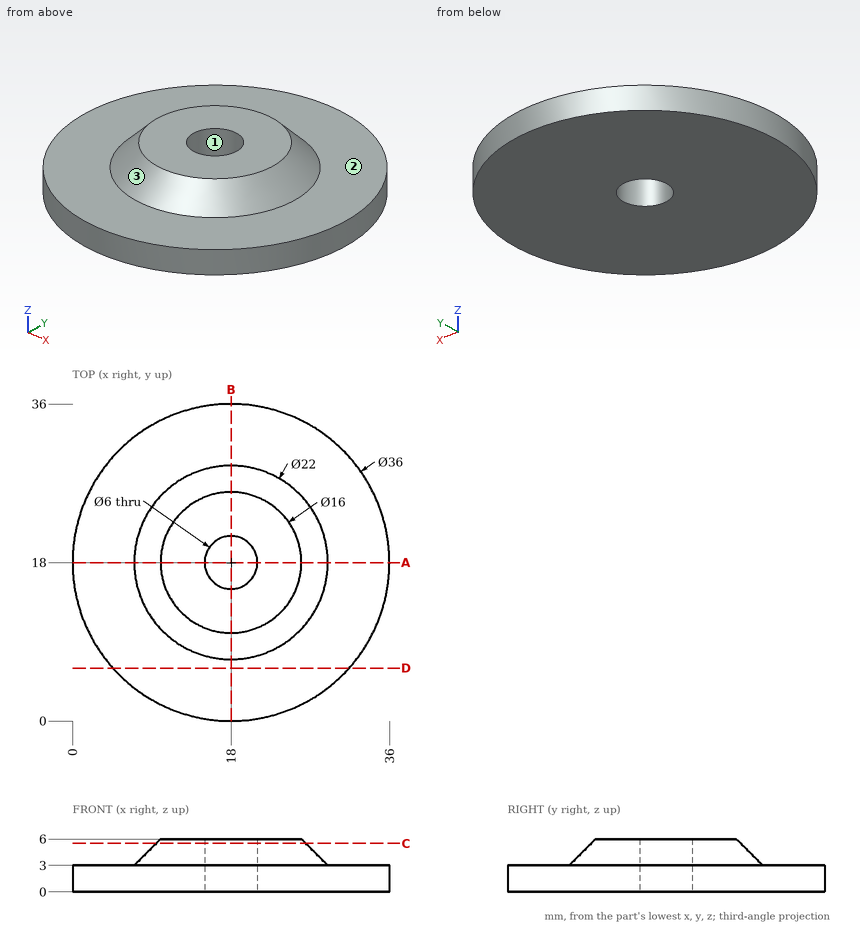
Input: dimensioned drawing with shaded views. Units: mm. Origin: part minimum x, y, z. Coordinates: 2 decimals unless noted, no trailing zeros. Loops run counter-clockwise (first coordinate to the right, second up) from the corner with the lowest first, then second, coordinate; pieces in that order, holes last.
Q1. Section A-A, the plane y = 18. Return the cut outline in (x, z).
Results are:
outline: (0, 0) - (15, 0) - (15, 6) - (10, 6) - (7, 3) - (0, 3) - close; (21, 0) - (36, 0) - (36, 3) - (29, 3) - (26, 6) - (21, 6) - close
Q2. Section D-D, the plane y = 6. Return the cut outline in (x, z), and give its area (3 significant figures).
Results are:
outline: (4.58, 0) - (31.42, 0) - (31.42, 3) - (4.58, 3) - close
area: 80.5 mm2
Q3. Section C-C, the plane z = 5.5. Return the cut outline in (x, y), and give its area (3 significant figures).
Results are:
outline: circle Ø17 at (18, 18); hole circle Ø6 at (18, 18)
area: 199 mm2
Q4. Line query: line 1 along Z through (x, y) = (28.5, 31); line 2 along Y through (x, z) = (18, 4.4); line 3 along Y through (x, z) = (18, 4). Output: solid intervals per line, ascending.
Results are:
line 1: z = 0 to 3
line 2: y = 8.4 to 15, 21 to 27.6
line 3: y = 8 to 15, 21 to 28
Q5. Contact query for flat-ended pins moving along their axis: pin 1 (2 mm diameter, centred on x = 14, y = 17, fed in from -Z); pin 2 (1.5 mm diameter, centred on x = 24, z = 3, fed in from +Y); pin 3 (5 mm diameter, centred on x = 31, y = 5, fed in from +Z). Output: stop coordinate, or through.
Results are:
pin 1: stops at z = 0
pin 2: stops at y = 35.22
pin 3: stops at z = 3
Q6. Mould query, pull axis X, two halves, no side actions, for the marked faces 1, 2 and 3. Classes: +X half, -X half, draft (parallel to the pull), parting line (faces both ways), or undercut.
Results are:
face 1: undercut
face 2: draft
face 3: parting line
